Check sheet for the drawn part. Datum: minimum x, y, z corner. Units: mm. A direction names the side the tool comes from. Give positions to 0.01 mm unless a question says otherwise; leave off trailing zeros. Order: outer loops, then holes, each group sorted by start corner. A loop starts at its lowest first (then second) coordinate and runs counter-clockwise, first axis right, second up.
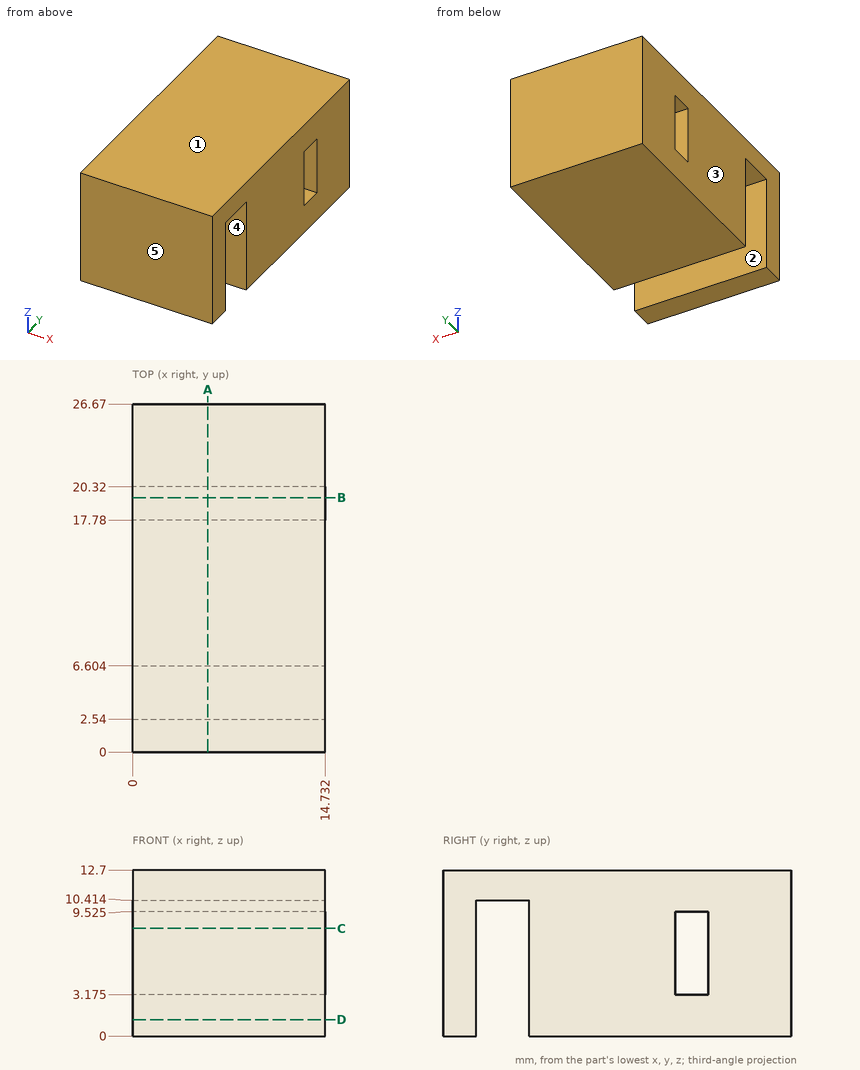
Item 1: Sectioned sample at D-D (z = 1.25). Enter the section's corners in (x, y), and give its area (3 significant figures).
Reported:
outline: (0, 0) - (14.73, 0) - (14.73, 2.54) - (0, 2.54) - close; (0, 6.6) - (14.73, 6.6) - (14.73, 26.67) - (0, 26.67) - close
area: 333 mm2
Item 2: Sectioned sample at A-A (x = 5.75). Enter the section's corners in (y, z) (3 decimals), and give its area (3 significant figures).
Reported:
outline: (0, 0) - (2.54, 0) - (2.54, 10.414) - (6.604, 10.414) - (6.604, 0) - (26.67, 0) - (26.67, 12.7) - (0, 12.7) - close; hole (17.78, 3.175) - (20.32, 3.175) - (20.32, 9.525) - (17.78, 9.525) - close
area: 280 mm2
Item 3: Set-up check for the marked faces 1 and 2: record each of +Z, -Z, +X, -X, +Y, -Y from which the full face is reachable in a straight line by a thin tool's end or side.
Reported:
face 1: +Z, +X, -X, +Y, -Y
face 2: -Z, +X, -X
Item 4: Sectioned sample at B-B (y = 19.5). Enter the section's corners in (x, z) (3 decimals).
Reported:
outline: (0, 0) - (14.732, 0) - (14.732, 3.175) - (0, 3.175) - close; (0, 9.525) - (14.732, 9.525) - (14.732, 12.7) - (0, 12.7) - close
Item 5: Draft check along Y on the marked faces 3, 4 and 5. Enter one of: released by +Y, released by -Y, zero draft, split by the parting line, or undercut.
Reported:
face 3: zero draft
face 4: undercut
face 5: released by -Y
Item 6: Scan lines: L1, parallel to Y at x = 6.5, z = 8.25; L2, parallel to Y at x = 6.75, z = 1.75; L3, parallel to Z at x = 0.5, y = 4.5. Record each from-to range of solid material in increasing order.
Reported:
L1: y = 0 to 2.54, 6.6 to 17.78, 20.32 to 26.67
L2: y = 0 to 2.54, 6.6 to 26.67
L3: z = 10.41 to 12.7
Item 7: Sectioned sample at C-C (z = 8.25). Enter the section's corners in (x, y).
Reported:
outline: (0, 0) - (14.73, 0) - (14.73, 2.54) - (0, 2.54) - close; (0, 6.6) - (14.73, 6.6) - (14.73, 17.78) - (0, 17.78) - close; (0, 20.32) - (14.73, 20.32) - (14.73, 26.67) - (0, 26.67) - close
